Source: CAD feature listing. Evaluate the final solid. Frame: model axes, mm. Face numbers are marked on the shaded views. Give positions to 0.01 mm unless a question says otherwise; leave off trailing zeros. Write each loop counter-clockwise with the first axis right and the second up, starting at its lowest first coordinate (ties: lowest second). Pieces come first, ordered by that corner, then holes. Notation, with made-up numbers: M -6.5,8.5 L 25.5,8.5 A9 ccw 25.5,19.5 Z; hole C 10.5,59 d4. An arc over 180 degrees is marked long. Return JSON: item names as keys, results as strings.
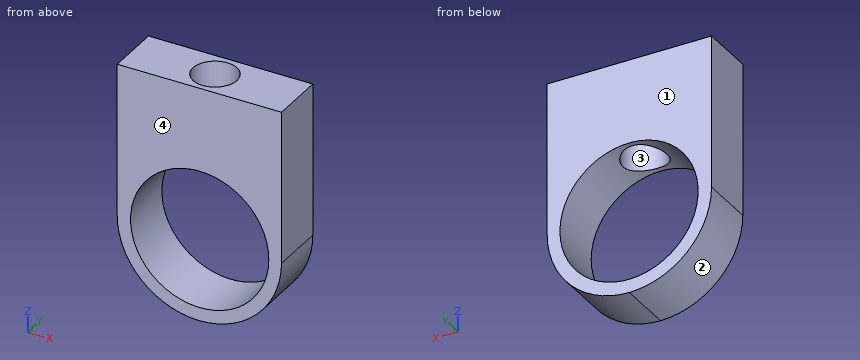
```python
from build123d import *

# Parameters (mm, degrees)
F0_R     = 12.569468
F1_DEPTH = 10
F2_R     = 4
F3_DEPTH = 25


with BuildPart() as f1:
    # F0 (on Front) → F1 (new body)
    with BuildSketch(Plane.XZ):
        with BuildLine():
            Line((9.299427, -18.636342), (9.299427, 9.197386))
            Line((9.299427, 9.197386), (-20.579568, 9.197386))
            Line((-20.579568, 9.197386), (-20.579568, -18.636342))
            ThreePointArc((-20.579568, -18.636342), (-16.207539, -29.221531), (-5.64007, -33.63622))
            ThreePointArc((-5.64007, -33.63622), (4.927398, -29.221531), (9.299427, -18.636342))
        make_face()
        with Locations((-5.579568, -18.636342)):
            Circle(F0_R, mode=Mode.SUBTRACT)
    extrude(amount=F1_DEPTH)

    # F2 (on face) → F3 (cut)
    with BuildSketch(Plane.XY.offset(9.197386)):
        with Locations((-5.64007, -5)):
            Circle(F2_R)
    extrude(amount=-F3_DEPTH, mode=Mode.SUBTRACT)


solid = f1.part
```
1) Contact query for a flat-ended pin moving along its axis: pin 1 Ø1.5 at (x, y) = (-6.5, -3.5) entering from -Z. Output: stop coordinate, or through.
Numbers:
{"pin 1": "stops at z = -33.64"}
2) Cut plane A-A, the plane x = -12.75. Return the cut outline in (y, z).
Numbers:
{"outline": "M -10,-31.81 L 0,-31.81 L 0,-28.96 L -10,-28.96 Z; M -10,-8.31 L 0,-8.31 L 0,9.2 L -10,9.2 Z"}
3) Cut plane B-B, the plane z = -7.5. Return the cut outline in (x, y), then the cut area to 3 significant figures.
Numbers:
{"outline": "M -20.58,-10 L -11.41,-10 L -11.41,0 L -20.58,0 Z; M 0.25,-10 L 9.3,-10 L 9.3,0 L 0.25,0 Z", "area": "182 mm²"}
4) Draft query along Y for the marked faces 1, 2, 3 and 4. Return one class per face: released by +Y, released by -Y, zero draft, split by the parting line, or undercut.
Numbers:
{"face 1": "released by +Y", "face 2": "zero draft", "face 3": "undercut", "face 4": "released by -Y"}
5) Line query: line 1 (X direction, y = -5, z = -0.75); line 2 (X direction, y = -9, z = -16); line 3 (Y direction, x = -5, z = 3). Output: solid intervals per line, ascending. Write a range as [from, to].
Numbers:
{"line 1": "x = [-20.58, -9.64], [-1.64, 9.3]", "line 2": "x = [-20.58, -17.87], [6.71, 9.3]", "line 3": "y = [-10, -8.95], [-1.05, 0]"}
6) Cut plane C-C, the plane x = -2.5. Return the cut outline in (y, z).
Numbers:
{"outline": "M -10,-33.29 L 0,-33.29 L 0,-30.82 L -10,-30.82 Z; M -10,-6.45 L -7.48,-6.45 L -7.48,9.2 L -10,9.2 Z; M -2.52,-6.45 L 0,-6.45 L 0,9.2 L -2.52,9.2 Z"}
7) Cut plane D-D, the plane y = -5. Return the cut outline in (x, z), then the cut area to 3 significant figures.
Numbers:
{"outline": "M -20.58,-18.64 A15 ccw -5.64,-33.64 A15 ccw 9.3,-18.64 L 9.3,9.2 L -1.64,9.2 L -1.64,-6.7 A12.57 cw long -9.64,-6.74 L -9.64,9.2 L -20.58,9.2 Z", "area": "563 mm²"}
